Drawing for the job (mm, zero at the part's lowest x, y, z). Round coordinates to 2 decimals unless told otherwise and drop trailing zeros. Loops run counter-clockwise (first coordinate to the right, second up) from the corner with the lowest first, then second, coordinate; pieces in that order, holes last.
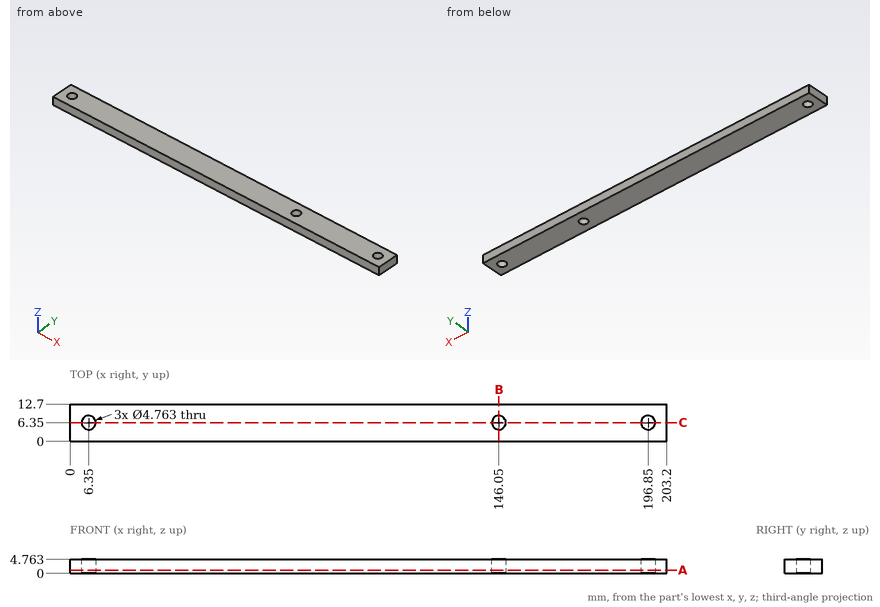
Q1. Slice it at A-A on z = 1.1. Give the cut face in (x, y).
Q2. Slice it at C-C on y = 6.35. Give the cut face in (x, z).
Q3. Probe line 1 (X direction, y = 6.35, z = 3.15); line 2 (Y direction, x = 146.05, z = 2); line 3 (X direction, y = 5, z = 1.1). List the from-to ranges inside material, lowest first.
Q4. Flat gauge pin, fed straight in: P1, Ø3, axis at x = 146.05, y = 6.35, coming from the +Z side. Where does the tip first touch, or does it go through?
Q5. Slice it at B-B on x = 146.05. Give the cut face in (y, z).
Reply:
1. outline: (0, 0) - (203.2, 0) - (203.2, 12.7) - (0, 12.7) - close; hole circle Ø4.76 at (6.35, 6.35); hole circle Ø4.76 at (146.05, 6.35); hole circle Ø4.76 at (196.85, 6.35)
2. outline: (0, 0) - (3.97, 0) - (3.97, 4.76) - (0, 4.76) - close; (8.73, 0) - (143.67, 0) - (143.67, 4.76) - (8.73, 4.76) - close; (148.43, 0) - (194.47, 0) - (194.47, 4.76) - (148.43, 4.76) - close; (199.23, 0) - (203.2, 0) - (203.2, 4.76) - (199.23, 4.76) - close
3. line 1: x = 0 to 3.97, 8.73 to 143.67, 148.43 to 194.47, 199.23 to 203.2
3. line 2: y = 0 to 3.97, 8.73 to 12.7
3. line 3: x = 0 to 4.39, 8.31 to 144.09, 148.01 to 194.89, 198.81 to 203.2
4. P1: passes through
5. outline: (0, 0) - (3.97, 0) - (3.97, 4.76) - (0, 4.76) - close; (8.73, 0) - (12.7, 0) - (12.7, 4.76) - (8.73, 4.76) - close
